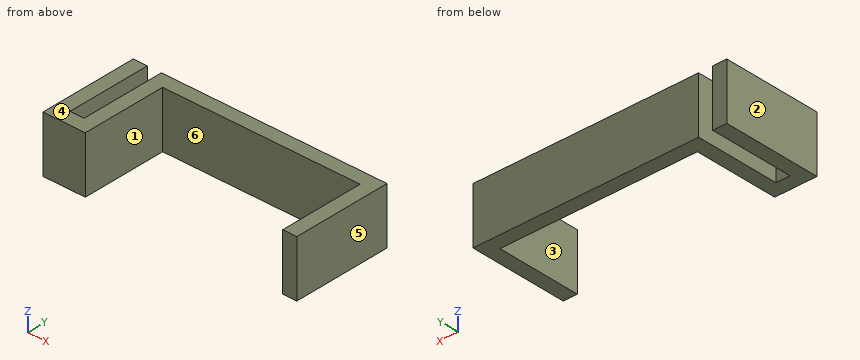
```python
from build123d import *

# Parameters (mm, degrees)
F0_W     = 6.35
F0_H     = 38.1
F1_DEPTH = 25.4


with BuildPart() as f1:
    # F0 (on Top) → F1 (new body)
    with BuildSketch(Plane.XY):
        with Locations((-60.325, 6.35)):
            Rectangle(F0_W, F0_H)
        Polygon((-63.5, -19.05), (-50.8, -19.05), (-50.8, -12.7), (-57.15, -12.7), (-63.5, -12.7), align=None)
        Polygon((-50.8, -19.05), (-44.45, -19.05), (-44.45, 19.05), (-50.8, 19.05), (-50.8, -12.7), align=None)
        Polygon((-44.45, 19.05), (44.45, 19.05), (44.45, 25.4), (-50.8, 25.4), (-50.8, 19.05), align=None)
        Polygon((44.45, 19.05), (44.45, -19.05), (50.8, -19.05), (50.8, 25.4), (44.45, 25.4), align=None)
    extrude(amount=F1_DEPTH)


solid = f1.part
```
For this review, take the finished solid that the model builds, in its own axes (mm). Face numbers are marked on the shaded views. A direction names the side the tool comes from. Give positions to 0.01 mm unless a question says otherwise; leave off trailing zeros. Write each loop counter-clockwise with the first axis right and the second up, starting at its lowest first coordinate (ties: lowest second). Pieces come first, ordered by that corner, then holes. Notation, with made-up numbers: M -24.75,68.25 L -6.75,68.25 A31 cw -6.75,94.25 Z; hole C -35.75,76.5 d1. An arc over 180 degrees is marked long. One line per item, written item: value.
1) For P1, Ø5, axis at x = -53, z = 14, coming from the +Y side; P2, Ø7.5, axis at x = -0.5, z = 10.5, coming from the -Y side, all flat-tipped, find the tip position at first contact; note any pin that passes through.
Results are:
P1: stops at y = 25.4
P2: stops at y = 19.05
2) The part is to be moulded in two halves that separate along X. For the marked faces 3, 4, 5 and 6, say which applies: +X half, -X half, draft (parallel to the pull), parting line (faces both ways), or undercut.
Results are:
face 3: undercut
face 4: draft
face 5: +X half
face 6: undercut
3) For line 1 (X direction, y = -11.5, z = 13.75); line 2 (Y direction, x = -37, z = 15); line 3 (X direction, y = 20.5, z = 17.5), list the stretches that pass through material, from the lowest coordinate up. Write a range as from..to.
Results are:
line 1: x = -63.5..-57.15, -50.8..-44.45, 44.45..50.8
line 2: y = 19.05..25.4
line 3: x = -63.5..-57.15, -50.8..50.8
4) Take a section at B-B, the plane y = -14. Write out the cut boundary in (x, z), then the cut area to 3 significant figures.
Results are:
outline: M -63.5,0 L -44.45,0 L -44.45,25.4 L -63.5,25.4 Z; M 44.45,0 L 50.8,0 L 50.8,25.4 L 44.45,25.4 Z
area: 645 mm²
5) Take a section at D-D, the plane x = 25.5. Write out the cut boundary in (y, z), then the cut area to 3 significant figures.
Results are:
outline: M 19.05,0 L 25.4,0 L 25.4,25.4 L 19.05,25.4 Z
area: 161 mm²
6) Take a section at A-A, the plane y = 0. Write out the cut boundary in (x, z).
Results are:
outline: M -63.5,0 L -57.15,0 L -57.15,25.4 L -63.5,25.4 Z; M -50.8,0 L -44.45,0 L -44.45,25.4 L -50.8,25.4 Z; M 44.45,0 L 50.8,0 L 50.8,25.4 L 44.45,25.4 Z
7) For the marked faces 1 and 2, list the 3-axis set-ups (+Z, -Z, +X, -X, +Y, -Y) from which the entire face can be reached by the end or side of a thin tool; tool diameter is ignored.
Results are:
face 1: +Z, -Z, -Y
face 2: +Z, -Z, -X, +Y, -Y
8) Take a section at C-C, the plane z = 7.5. Write out the cut boundary in (x, y), then the cut area to 3 significant figures.
Results are:
outline: M -63.5,-19.05 L -44.45,-19.05 L -44.45,19.05 L 44.45,19.05 L 44.45,-19.05 L 50.8,-19.05 L 50.8,25.4 L -50.8,25.4 L -50.8,-12.7 L -57.15,-12.7 L -57.15,25.4 L -63.5,25.4 Z
area: 1,450 mm²
